Design review of the part built by this model. Coordinates are the model's own, in mm. Face numbers are marked on the shaded views. Coordinates: 2 decimals unless noted, no trailing zeros. Order: outer loops, then holes, each group sorted by start corner. A loop starts at its lowest first (then second) coordinate and runs counter-clockwise, first axis right, second up. Notation, with made-up numbers: M -26.5,8.25 L -3.5,8.25 A22 cw -3.5,37.25 Z; hole C 17.5,-17 d6. An arc over 180 degrees is marked long. Use CSV: the item, a comma, the result in double quotes.
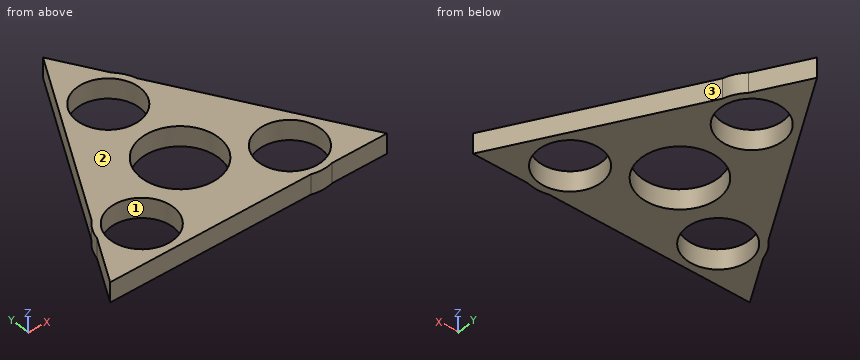
```python
from build123d import *

# Parameters (mm, degrees)
F0_R     = 11.05
F0_R_2   = 13.55
F1_DEPTH = 7


with BuildPart() as f1:
    # F0 (on Top) → F1 (new body)
    with BuildSketch(Plane.XY):
        with BuildLine():
            ThreePointArc((9.3366927058, 39.8345466227), (-12.4522023386, 24.671969793), (13.55, 30.0147365779))
            ThreePointArc((13.55, 30.0147365779), (13.4383509122, 31.7506008471), (13.1052435777, 33.4578588192))
            Line((13.1052435777, 33.4578588192), (9.3366927058, 39.8345466227))
        make_face()
        with Locations((0, 30.0147365779)):
            Circle(F0_R, mode=Mode.SUBTRACT)
        with BuildLine():
            ThreePointArc((13.1052435777, 33.4578588192), (13.4383509122, 31.7506008471), (13.55, 30.0147365779))
            ThreePointArc((13.55, 30.0147365779), (-12.4522023386, 24.671969793), (9.3366927058, 39.8345466227))
            Line((9.3366927058, 39.8345466227), (-0.5756262346, 56.6069786372))
            Line((-0.5756262346, 56.6069786372), (-35.4637109435, -5.2654817113))
            ThreePointArc((-35.4637109435, -5.2654817113), (-20.7479078997, -2.5094129528), (-12.4766616182, -14.9888864664))
            ThreePointArc((-12.4766616182, -14.9888864664), (-27.5580450783, -28.4520719995), (-39.2305161863, -11.9457426075))
            Line((-39.2305161863, -11.9457426075), (-48.735268414, -28.8019962609))
            Line((-48.735268414, -28.8019962609), (22.3233113272, -28.0794142811))
            ThreePointArc((22.3233113272, -28.0794142811), (17.7660584346, -4.2357986208), (39.5109500096, -15.0268250814))
            ThreePointArc((39.5109500096, -15.0268250814), (36.8347466684, -23.1115666494), (29.8632679104, -28.002741812))
            Line((29.8632679104, -28.002741812), (49.3108946486, -27.8049823764))
            Line((49.3108946486, -27.8049823764), (13.1052435777, 33.4578588192))
        make_face()
        Circle(F0_R_2, mode=Mode.SUBTRACT)
        with BuildLine():
            Line((9.3366927058, 39.8345466227), (13.1052435777, 33.4578588192))
            ThreePointArc((13.1052435777, 33.4578588192), (11.6651473576, 36.9087076487), (9.3366927058, 39.8345466227))
        make_face()
        with BuildLine():
            Line((22.3233113272, -28.0794142811), (29.8632679104, -28.002741812))
            ThreePointArc((29.8632679104, -28.002741812), (36.8347466684, -23.1115666494), (39.5109500096, -15.0268250814))
            ThreePointArc((39.5109500096, -15.0268250814), (17.7660584346, -4.2357986208), (22.3233113272, -28.0794142811))
        make_face()
        with Locations((25.9609500096, -15.0268250814)):
            Circle(F0_R, mode=Mode.SUBTRACT)
        with BuildLine():
            ThreePointArc((22.3233113272, -28.0794142811), (26.0987304111, -28.5761245674), (29.8632679104, -28.002741812))
            Line((29.8632679104, -28.002741812), (22.3233113272, -28.0794142811))
        make_face()
        with BuildLine():
            Line((-39.2305161863, -11.9457426075), (-35.4637109435, -5.2654817113))
            ThreePointArc((-35.4637109435, -5.2654817113), (-37.8295893773, -8.3335580513), (-39.2305161863, -11.9457426075))
        make_face()
        with BuildLine():
            ThreePointArc((-12.4766616182, -14.9888864664), (-20.7479078997, -2.5094129528), (-35.4637109435, -5.2654817113))
            Line((-35.4637109435, -5.2654817113), (-39.2305161863, -11.9457426075))
            ThreePointArc((-39.2305161863, -11.9457426075), (-27.5580450783, -28.4520719995), (-12.4766616182, -14.9888864664))
        make_face()
        with Locations((-26.0266616182, -14.9888864664)):
            Circle(F0_R, mode=Mode.SUBTRACT)
    extrude(amount=F1_DEPTH)


solid = f1.part
```
(1) Add section B-B on y = 11. State the section outline as (x, z) points, and give its area (3 significant figures).
The answers:
outline,"M -26.29,0 L -7.91,0 L -7.91,7 L -26.29,7 Z; M 7.91,0 L 26.38,0 L 26.38,7 L 7.91,7 Z"
area,"258 mm2"
(2) Clearance check with flat-ended pins moving along their axes: P1, Ø1, axis at x = 11, z = 3.5, coming from the -Y side; P2, Ø4, axis at x = -8.5, z = 1.5, coming from the -Y side; P3, Ø21.5, axis at x = 0, y = 0, coming from the -Z side; P4, Ø2, axis at x = 24.5, z = 5, coming from the -Y side. State where each tip first meets the part, or that it passes through.
The answers:
P1,"stops at y = -28.2"
P2,"stops at y = -28.41"
P3,"passes through"
P4,"stops at y = -28.57"
(3) Wall thickness on probe 1 along X at (y, z) = (-20, 1); probe 2 along Y at (x, z) = (0, 2.75); probe 3 along Y at (x, z) = (4, 0.75): over which ranges is each line inside the solid? List them lowest first.
The answers:
probe 1,"x = -43.77 to -35.88, -16.18 to 16.09, 35.83 to 44.7"
probe 2,"y = -28.31 to -13.55, 13.55 to 18.96, 41.06 to 55.63"
probe 3,"y = -28.27 to -12.95, 12.95 to 19.71, 40.32 to 48.86"
(4) Add section C-C on z = 4.25. State the section outline as (x, y) points, and give its area (3 significant figures).
The answers:
outline,"M -48.74,-28.8 L 22.32,-28.08 A13.55 ccw 29.86,-28 L 49.31,-27.8 L 13.11,33.46 A13.55 ccw 9.34,39.83 L -0.58,56.61 L -35.46,-5.27 A13.55 ccw -39.23,-11.95 Z; hole C -26.03,-14.99 d22.1; hole C 0,0 d27.1; hole C 0,30.01 d22.1; hole C 25.96,-15.03 d22.1"
area,"2,440 mm2"
(5) The part is to be moulded in two halves that separate along Y. For the marked faces 1, 2 and 3, say which applies: pulls with the +Y half, pulls with the -Y half, needs draft (parallel to the pull), parting line crosses it, or undercut.
The answers:
face 1,"undercut"
face 2,"needs draft"
face 3,"pulls with the +Y half"
(6) Add section A-A on x = -32.5. State the section outline as (y, z) points, and give its area (3 significant figures).
The answers:
outline,"M -28.64,0 L -23.94,0 L -23.94,7 L -28.64,7 Z; M -6.03,0 L -0.01,0 L -0.01,7 L -6.03,7 Z"
area,"75.0 mm2"
